Design review of the part built by this model. Coordinates are the model's own, in mm. Coordinates: 2 decimals unless noted, no trailing zeros. Order: outer loops, then holes, each group sorted by start corner. A loop starts at its lowest first (then second) coordinate and runs counter-clockwise, first axis right, second up.
from build123d import *

# Parameters (mm, degrees)
SKETCH1_R           = 80.518
SKETCH1_R_2         = 79.375
BOSS_EXTRUDE1_DEPTH = 838.2
SKETCH3_W           = 3.2004
SKETCH3_H           = 204.978
CUT_EXTRUDE1_DEPTH  = 1.159132
CIRPATTERN1_COUNT   = 4


with BuildPart() as part:
    # Sketch1 → Boss-Extrude1 (new body)
    with BuildSketch(Plane.XY):
        Circle(SKETCH1_R)
        Circle(SKETCH1_R_2, mode=Mode.SUBTRACT)
    extrude(amount=BOSS_EXTRUDE1_DEPTH)

    # Sketch3 → Cut-Extrude1 (cut)
    with BuildSketch(Plane(origin=(0, 80.518, 0), x_dir=(1, 0, 0), z_dir=(0, 1, 0))):
        with Locations((0, -127.889)):
            Rectangle(SKETCH3_W, SKETCH3_H)
    cut_extrude1 = extrude(amount=-CUT_EXTRUDE1_DEPTH, mode=Mode.SUBTRACT)

    # CirPattern1: Cut-Extrude1 ×4 about axis
    cirpattern1_axis = Axis((0, 0, 0), (0, 0, 1))
    for i in range(1, CIRPATTERN1_COUNT):
        add(cut_extrude1.rotate(cirpattern1_axis, i * 360 / CIRPATTERN1_COUNT), mode=Mode.SUBTRACT)


solid = part.part
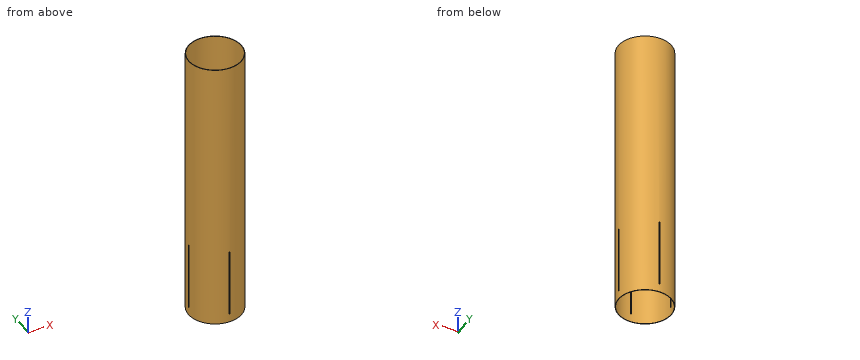
1. To check wall thickness, follow line 1 (X direction, y = -1, z = 725); line 2 (Y direction, x = 0, z = 345.5) (3 decimals); line 3 (X direction, y = -18, z = 473.5). State the ranges of each line that lie inside material, in increasing order.
2. Insertion check: pin 1 (1 mm diameter, centred on x = -60, z = 202, fed in from -Y); pin 2 (0.6 mm diameter, centred on x = -80, y = 0.5, fed in from -Z); pin 3 (8 mm diameter, centred on y = 15, z = 516, fed in from +X); pin 4 (4 mm diameter, centred on x = -28.5, z = 511.5, fed in from +Y). Each pin has a flat end and moves straight along its axis. Give the tip position at first contact, or say it passes through.
3. Add section A-A (z = 162.5). Give the boundary of the cut face in (x, y) (3 decimals).
4. Add section D-D (z = 451.5). Give the boundary of the cut face in (x, y) (3 decimals).
5. Add section C-C (y = 21). Give the boundary of the cut face in (x, z).
6. Add section B-B (x = 17.5). Give the boundary of the cut face in (y, z).
Solution:
1. line 1: x = -80.51 to -79.37, 79.37 to 80.51
1. line 2: y = -80.518 to -79.375, 79.375 to 80.518
1. line 3: x = -78.48 to -77.31, 77.31 to 78.48
2. pin 1: stops at y = -54.25
2. pin 2: stops at z = 0
2. pin 3: stops at x = 79.76
2. pin 4: stops at y = 76.03
3. outline: (-80.502, -1.6) arc R80.518 ccw to (-1.6, -80.502) - (-1.6, -79.359) arc R79.375 cw to (-79.359, -1.6) - close; (-80.502, 1.6) - (-79.359, 1.6) arc R79.375 cw to (-1.6, 79.359) - (-1.6, 80.502) arc R80.518 ccw to start; (1.6, -80.502) arc R80.518 ccw to (80.502, -1.6) - (79.359, -1.6) arc R79.375 cw to (1.6, -79.359) - close; (1.6, 79.359) arc R79.375 cw to (79.359, 1.6) - (80.502, 1.6) arc R80.518 ccw to (1.6, 80.502) - close
4. outline: circle Ø161.036 at (0, 0); hole circle Ø158.75 at (0, 0)
5. outline: (-77.73, 0) - (-76.55, 0) - (-76.55, 838.2) - (-77.73, 838.2) - close; (76.55, 0) - (77.73, 0) - (77.73, 838.2) - (76.55, 838.2) - close
6. outline: (-78.59, 0) - (-77.42, 0) - (-77.42, 838.2) - (-78.59, 838.2) - close; (77.42, 0) - (78.59, 0) - (78.59, 838.2) - (77.42, 838.2) - close
